Source: CAD feature listing. Evaluate the final solid. Frame: model axes, mm. Face numbers are marked on the shaded views. A direction names the side the tool comes from. Give positions to 0.01 mm unless a question says otherwise; leave off trailing zeros. Order: outer loops, then holes, each group sorted by start corner. A loop starts at its lowest first (then second) coordinate and runs counter-clockwise, first axis right, second up. Notation, with made-up numbers: (-16.75, 1.25) - (4.25, 1.25) arc R35 cw to (4.25, 36.25) - close; hole circle Ø8 at (53, 34.25). An arc over 180 degrees is marked (long way). Write each question's results on one line, items separated by ' | '. Start each with the question number.
Item 1: Set-up query: the marked faces 1 and 2. Return all of +Z, -Z, +X, -X, +Y, -Y with unobstructed straight access to the full face (end or side cutting, diameter ignored); none if empty.
Item 2: Section B-B on x = 48. Output: boundary loops of the cut face in (y, z), and give its area (3 significant figures).
Item 3: Contact query for flat-ended pins moving along their axis: pin 1 Ø13.5 at (y, z) = (-29, 19.5) entering from -X; pin 2 Ø4 at (x, z) = (31, 27.5) entering from -Y; pin 3 Ø8.5 at (x, y) = (34.5, 12.5) entering from +Z. Output: stop coordinate, or through.
Item 4: Section D-D on x = 4. Output: boundary loops of the cut face in (y, z), and give its area (3 significant figures).
Item 5: Line query: line 1 along X through (y, z) = (5, 5); line 2 along Y through (x, z) = (48, 4); line 3 along Y through (x, z) = (3, 3.4). Output: solid intervals per line, ascending.
Item 6: Section A-A on y = 6. Output: boundary loops of the cut face in (x, z), and give its area (3 significant figures).
Item 7: Section C-C on z = 21.5. Output: boundary loops of the cut face in (x, y).
```python
from build123d import *

# Parameters (mm, degrees)
ESQUISSE1_W             = 51
ESQUISSE1_H             = 28
BOSS_EXTRU_1_DEPTH      = 6
ESQUISSE2_R             = 1.75
ENL_V_MAT_EXTRU_1_DEPTH = 59.489315264
BOSS_EXTRU_2_DEPTH      = 51
ESQUISSE4_W             = 17.5
ESQUISSE4_H             = 30
ENL_V_MAT_EXTRU_2_DEPTH = 4.914913
CONG_1_R                = 8


with BuildPart() as part:
    # Esquisse1 → Boss.-Extru.1 (new body)
    with BuildSketch(Plane.XY):
        with Locations((25.5, 14)):
            Rectangle(ESQUISSE1_W, ESQUISSE1_H)
    extrude(amount=BOSS_EXTRU_1_DEPTH)

    # Esquisse2 → Enlèv. mat.-Extru.1 (cut, through all)
    with BuildSketch(Plane.XY.offset(6)):
        with Locations((3, 6)):
            Circle(ESQUISSE2_R)
        with Locations((3, 22)):
            Circle(ESQUISSE2_R)
        with Locations(Location((48, 22, 0), (0, 0, 180))):
            Circle(ESQUISSE2_R)
        with Locations(Location((48, 6, 0), (0, 0, 180))):
            Circle(ESQUISSE2_R)
    extrude(amount=-ENL_V_MAT_EXTRU_1_DEPTH, mode=Mode.SUBTRACT)

    # Esquisse3 → Boss.-Extru.2 (add)
    with BuildSketch(Plane.ZY):
        Polygon((0, 0), (28.678821818, -40.957602214), (32.704882248, -38.138524352), (6, 0), align=None)
    extrude(amount=-BOSS_EXTRU_2_DEPTH)

    # Esquisse4 → Enlèv. mat.-Extru.2 (cut)
    with BuildSketch(Plane(origin=(0, 0, 0), x_dir=(-1, 0, 0), z_dir=(0, -0.5735764363510419, -0.8191520442889949))):
        with Locations((-8.75, -35)):
            Rectangle(ESQUISSE4_W, ESQUISSE4_H)
        with Locations((-42.25, -35)):
            Rectangle(ESQUISSE4_W, ESQUISSE4_H)
    extrude(amount=-ENL_V_MAT_EXTRU_2_DEPTH, mode=Mode.SUBTRACT)

    # Congé1
    cong_1_edges = [part.edges().sort_by_distance(p)[0] for p in [
        (33.5, -14.973501955, 13.484558942),
        (17.5, -14.973501955, 13.484558942),
        (33.5, -39.548063283, 30.691852033),
        (17.5, -39.548063283, 30.691852033),
        (0, -14.973501955, 13.484558942),
        (51, -14.973501955, 13.484558942),
    ]]
    fillet(cong_1_edges, radius=CONG_1_R - 0.0001)  # a hair under: the kernel refuses the full size


solid = part.part
```
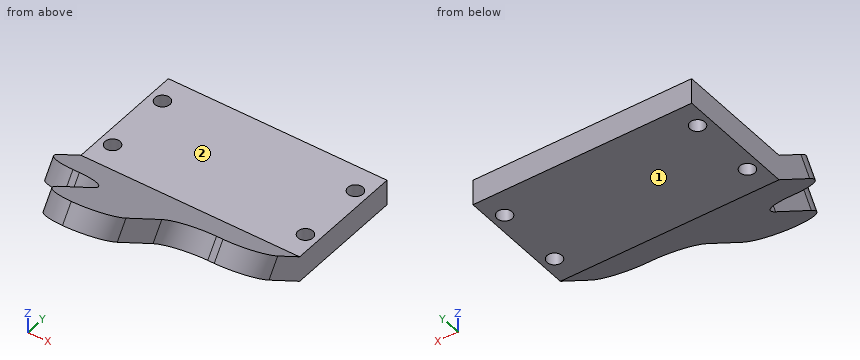
Evaluation:
1) face 1: -Z, +X, -X, +Y, -Y | face 2: +Z, +X, -X, +Y
2) outline: (-14.95, 10.46) - (0, 0) - (4.25, 0) - (4.25, 6) - (0, 6) - (-12.13, 14.49) - close; (7.75, 0) - (20.25, 0) - (20.25, 6) - (7.75, 6) - close; (23.75, 0) - (28, 0) - (28, 6) - (23.75, 6) - close | area: 207 mm^2
3) pin 1: stops at x = 17.5 | pin 2: stops at y = -40.25 | pin 3: stops at z = 6
4) outline: (-15.51, 10.86) - (0, 0) - (4.56, 0) - (4.56, 6) - (0, 6) - (-12.69, 14.88) - close; (7.44, 0) - (20.56, 0) - (20.56, 6) - (7.44, 6) - close; (23.44, 0) - (28, 0) - (28, 6) - (23.44, 6) - close | area: 218 mm^2
5) line 1: x = 0 to 1.56, 4.44 to 46.56, 49.44 to 51 | line 2: y = -5.71 to 4.25, 7.75 to 20.25, 23.75 to 28 | line 3: y = -4.86 to 4.25, 7.75 to 20.25, 23.75 to 28
6) outline: (0, 0) - (1.25, 0) - (1.25, 6) - (0, 6) - close; (4.75, 0) - (46.25, 0) - (46.25, 6) - (4.75, 6) - close; (49.75, 0) - (51, 0) - (51, 6) - (49.75, 6) - close | area: 264 mm^2
7) outline: (17.5, -30.71) - (33.5, -30.71) - (33.5, -22.14) - (17.5, -22.14) - close
